from build123d import *

# Parameters (mm, degrees)
F0_R      = 2
F0_R_2    = 4.25
F1_DEPTH  = 6
F4_R      = 1.6
F5_DEPTH  = 15
F8_DEPTH  = 3.5
F11_R     = 3.25
F12_DEPTH = 2.5


with BuildPart() as f1:
    # F0 (on Front) → F1 (new body)
    with BuildSketch(Plane.XZ):
        with BuildLine():
            add(Edge.make_bspline(
                [(10, -12.5), (5, -12.5), (0, -3), (-5, -12.5), (-10, -12.5)],
                knots=[0, 0, 0, 0, 0.5, 1, 1, 1, 1], degree=3))
            ThreePointArc((10, -12.5), (13.8302222156, -10.7139380484), (14.9240387651, -6.6317591117))
            Line((14.9240387651, -6.6317591117), (13.3399263315, 2.3521889329))
            Line((13.3399263315, 2.3521889329), (13.079454065, 3.8294005624))
            ThreePointArc((13.079454065, 3.8294005624), (11.6401444567, 6.0886640956), (9.0248583076, 6.6684590761))
            Line((9.0248583076, 6.6684590761), (3.5557645771, 5.7041102914))
            ThreePointArc((3.5557645771, 5.7041102914), (1.8492439019, 6.4622467406), (0, 6.7216319406))
            ThreePointArc((0, 6.7216319406), (-1.8492439019, 6.4622467406), (-3.5557645771, 5.7041102914))
            Line((-3.5557645771, 5.7041102914), (-9.0248583076, 6.6684590761))
            ThreePointArc((-9.0248583076, 6.6684590761), (-11.6401444567, 6.0886640956), (-13.079454065, 3.8294005624))
            Line((-13.079454065, 3.8294005624), (-13.3399263315, 2.3521889329))
            Line((-13.3399263315, 2.3521889329), (-14.9240387651, -6.6317591117))
            ThreePointArc((-14.9240387651, -6.6317591117), (-13.8302222156, -10.7139380484), (-10, -12.5))
        make_face()
        with Locations((-10, -7.5)):
            Circle(F0_R, mode=Mode.SUBTRACT)
        with Locations((10, -7.5)):
            Circle(F0_R, mode=Mode.SUBTRACT)
        Circle(F0_R_2, mode=Mode.SUBTRACT)
    extrude(amount=-F1_DEPTH)


with BuildPart() as f5:
    # F4 (on line) → F5 (new body)
    with BuildSketch(Plane(origin=(0, 0, 0), x_dir=(0, 1, 0), z_dir=(0.984807753, 0, 0.1736481777))):
        with Locations((3, 0)):
            Circle(F4_R)
    extrude(amount=F5_DEPTH)


with BuildPart() as f8:
    # F7 (on offset) → F8 (new body)
    with BuildSketch(Plane(origin=(5.9088465181, 0, 1.041889066), x_dir=(0, 1, 0), z_dir=(0.984807753, 0, 0.1736481777))):
        Polygon((1.2679491924, -3), (4.7320508076, -3), (6.4641016151, 0), (4.7320508076, 3), (1.2679491924, 3), (-12.080499812, 3), (-12.080499812, -3), align=None)
    extrude(amount=F8_DEPTH)


with BuildPart() as f9_1:
    # F9: instance of F5
    add(f5.part.mirror(Plane.YZ))


with BuildPart() as f9_2:
    # F9: instance of F8
    add(f8.part.mirror(Plane.YZ))


with BuildPart() as f1_1:
    add(f1.part)

    # F10: cut F8, F5, F9_1, F9_2
    add(f8.part, mode=Mode.SUBTRACT)
    add(f5.part, mode=Mode.SUBTRACT)
    add(f9_1.part, mode=Mode.SUBTRACT)
    add(f9_2.part, mode=Mode.SUBTRACT)

    # F11 (on face) → F12 (cut)
    with BuildSketch(Plane.XZ):
        with Locations((-10, -7.5)):
            Circle(F11_R)
        with Locations((10, -7.5)):
            Circle(F11_R)
    extrude(amount=-F12_DEPTH, mode=Mode.SUBTRACT)


solid = f1_1.part
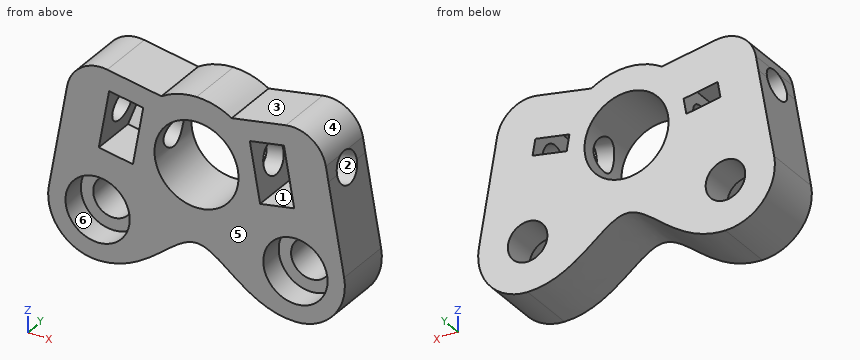
Can you work these out from the model? Positions are in its coordinate system, mm. Face numbers are marked on the shaded views. A direction names the side the tool comes from. Round coordinates to 2 decimals unless told otherwise and drop trailing zeros. Use CSV: the item, a comma, the result in double quotes.
(1) I'm going to push flat-ended pins straight in: pin 1 (7 mm diameter, centred on x = -10.5, z = -7.5, fed in from -Y); pin 2 (7 mm diameter, centred on x = 0, z = 0, fed in from +Y); pin 3 (1.5 mm diameter, centred on x = -8.5, y = 5.5, fed in from -Z); pin 4 (1.5 mm diameter, centred on x = 7, y = 3.5, fed in from -Z). Where does each tip first touch, or does it pass through?
Check values:
pin 1,"y = 0"
pin 2,"through"
pin 3,"z = -12.46"
pin 4,"z = -12.16"
(2) On a 3-axis mill with a long thin cutter (end or side, diameter ignored), from which of +Z, -Z, +X, -X, +Y, -Y can I reach the whole of each face in a straight line? I mean the marked faces 1, 2 and 3. Say none if no direction works.
Check values:
face 1,"-Y"
face 2,"none"
face 3,"+Z, +Y, -Y"
(3) We'd pull the mould along Z, two halves only. Please class the marked faces 4, 5 and 6: +Z half, -Z half, draft (parallel to the pull), parting line (faces both ways), or undercut.
Check values:
face 4,"+Z half"
face 5,"draft"
face 6,"undercut"
(4) Imagine slicing it at A-A (y = 1). Count the separate pieces of the cut face and the enclosed holes in it, plus the area to 3 significant figures.
Check values:
separate pieces,"1"
enclosed holes,"5"
area,"315 mm^2"
(5) I need wall thicknesses on line 1 along Z through (x, y) = (0, 3.75); line 2 along Z through (x, y) = (-10, 1.6); line 3 along X through (y, z) = (2.25, -9). Which ranges of each line are inside material? Lowest first, please.
Check values:
line 1,"-7.75 to -4.25, 4.25 to 6.72"
line 2,"-12.5 to -10.75, -4.25 to 0.98, 2.55 to 6.7"
line 3,"-14.77 to -12.88, -7.12 to -2.62, 2.62 to 7.12, 12.88 to 14.77"
